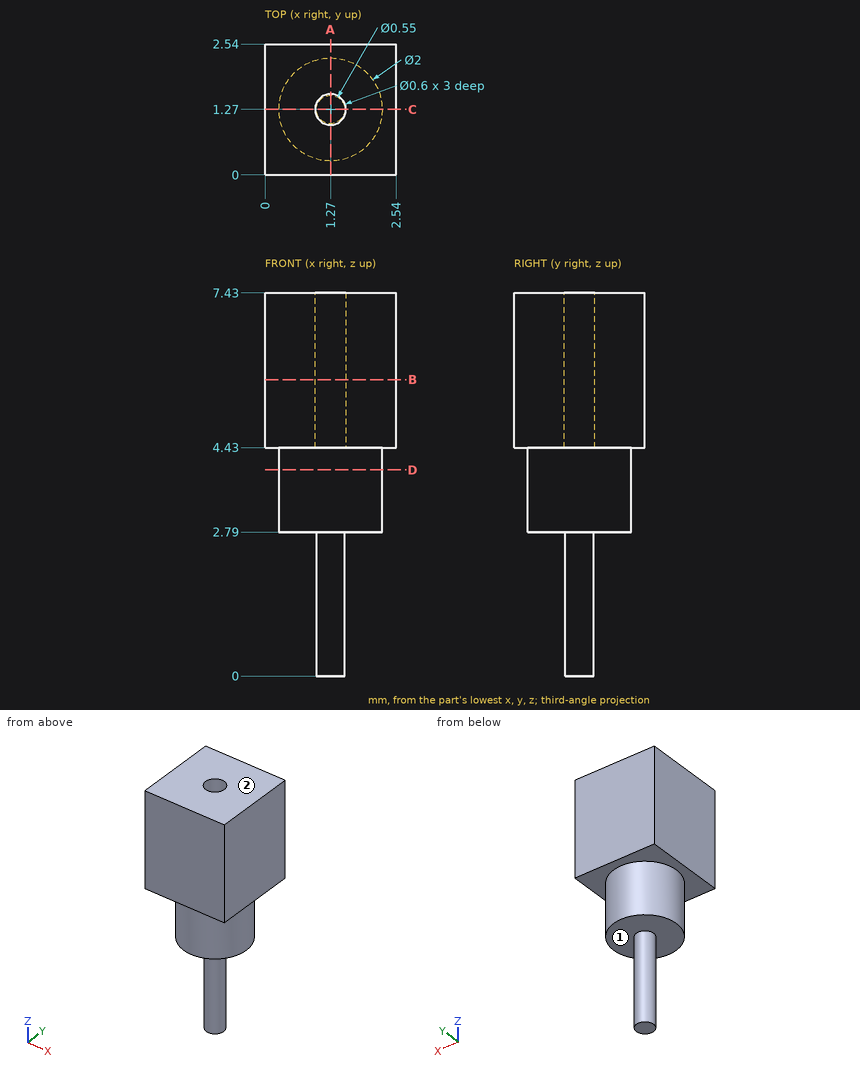
Could you check a few things on this drawing? It's one solid part, dimensions in mm from its lowest x, y, z. A direction names the side the tool comes from. Coordinates: 2 decimals unless noted, no trailing zeros. Loops run counter-clockwise (first coordinate to the right, second up) from the corner with the lowest first, then second, coordinate; pieces in that order, holes last. Notation, with made-up numbers: (63.25, 15) - (78.25, 15) arc R13 ccw to (78.25, 30) - close; hole circle Ø7 at (88.25, 85.25). An arc over 180 degrees is marked (long way). Answer as a JSON object with one key per item and string values. Group by question number.
Item 1: If we section it at D-D (z = 4): List the corners of the cut face in (x, y) for me.
Item 2: For pin 1 (1 mm diameter, centred on x = 1.5, z = 2, fed in from -Y) (3 decimals), with a flat end and sliding along its axis, tell me the tip position at first contact or that it passes through.
Item 3: If I drill on L1, parallel to Y at x = 1.27, z = 5.95; L2, parallel to Z at x = 2.35, y = 0.55; L3, parallel to Z at x = 1.5, y = 1.55, over which ranges is the centre line in solid material (lowest first)? Write a range as from..to.
Item 4: If we section it at A-A (x = 1.27): List the corners of the cut face in (y, z) for me (3 decimals), plus the area to 3 significant figures.
Item 5: On a 3-axis mill with a long thin cutter (end or side, diameter ignored), from which of +Z, -Z, +X, -X, +Y, -Y can I reach the whole of each face in a straight line? I mean the marked faces 1 and 2. Say none if no direction works.
Item 6: If we section it at B-B (z = 5.75): List the corners of the cut face in (x, y) for me, plus the area to 3 significant figures.
Returned:
{
 "1": {"outline": "circle Ø2 at (1.27, 1.27)"},
 "2": {"pin 1": "stops at y = 0.995"},
 "3": {"L1": "y = 0..0.97, 1.57..2.54", "L2": "z = 4.43..7.43", "L3": "z = 2.79..7.43"},
 "4": {"outline": "(0, 4.43) - (0.27, 4.43) - (0.27, 2.79) - (0.995, 2.79) - (0.995, 0) - (1.545, 0) - (1.545, 2.79) - (2.27, 2.79) - (2.27, 4.43) - (2.54, 4.43) - (2.54, 7.43) - (1.57, 7.43) - (1.57, 4.43) - (0.97, 4.43) - (0.97, 7.43) - (0, 7.43) - close", "area": "10.6 mm²"},
 "5": {"face 1": "-Z", "face 2": "+Z, +X, -X, +Y, -Y"},
 "6": {"outline": "(0, 0) - (2.54, 0) - (2.54, 2.54) - (0, 2.54) - close; hole circle Ø0.6 at (1.27, 1.27)", "area": "6.17 mm²"}
}
